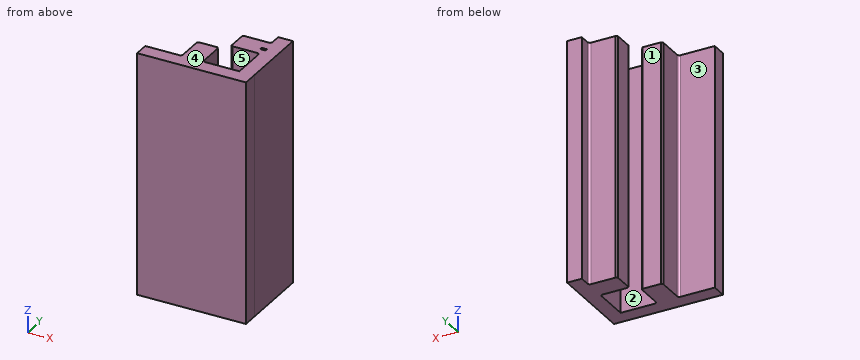
from build123d import *

# Parameters (mm, degrees)
BOSS_EXTRUDE1_DEPTH = 66.675
CUT_EXTRUDE1_REACH  = 75.8
CUT_EXTRUDE2_REACH  = 75.8
SKETCH5_W           = 1.489310624
SKETCH5_H           = 0.739469686
CUT_EXTRUDE3_DEPTH  = 2.54


with BuildPart() as part:
    # Sketch1 → Boss-Extrude1 (new body)
    with BuildSketch(Plane(origin=(0, 0, -3683), x_dir=(-1, 0, 0), z_dir=(0, 0, -1))):
        with BuildLine():
            Line((7.945265893, 3.588862728), (-1.198734107, 3.588862728))
            ThreePointArc((-1.198734107, 3.588862728), (-1.647746913, 3.774849922), (-1.833734107, 4.223862728))
            Line((-1.833734107, 4.223862728), (-1.833734107, 5.747862728))
            ThreePointArc((-1.833734107, 5.747862728), (-1.647746913, 6.196875535), (-1.198734107, 6.382862728))
            Line((-1.198734107, 6.382862728), (1.621629442, 6.382862728))
            Line((1.621629442, 6.382862728), (1.621629442, 6.890862686))
            Line((1.621629442, 6.890862686), (-2.214734107, 11.462862728))
            Line((-2.214734107, 11.462862728), (-7.294734107, 11.462862728))
            Line((-7.294734107, 11.462862728), (-11.131097656, 6.890862686))
            Line((-11.131097656, 6.890862686), (-11.131097656, 6.382862728))
            Line((-11.131097656, 6.382862728), (-8.310734107, 6.382862728))
            ThreePointArc((-8.310734107, 6.382862728), (-7.861721301, 6.196875535), (-7.675734107, 5.747862728))
            Line((-7.675734107, 5.747862728), (-7.675734107, 4.223862728))
            ThreePointArc((-7.675734107, 4.223862728), (-7.861721301, 3.774849922), (-8.310734107, 3.588862728))
            Line((-8.310734107, 3.588862728), (-17.454734107, 3.588862728))
            Line((-17.454734107, 3.588862728), (-17.727921752, 3.588862728))
            Line((-17.727921752, 3.588862728), (-17.727921752, 3.858842754))
            Line((-17.727921752, 3.858842754), (-17.728361466, 13.002372481))
            ThreePointArc((-17.728361466, 13.002372481), (-17.542256287, 13.451715967), (-17.092921752, 13.637842754))
            Line((-17.092921752, 13.637842754), (-15.568921752, 13.637842754))
            ThreePointArc((-15.568921752, 13.637842754), (-15.119908946, 13.45185556), (-14.933921752, 13.002842754))
            Line((-14.933921752, 13.002842754), (-14.933921752, 10.182479205))
            Line((-14.933921752, 10.182479205), (-14.425921794, 10.182479205))
            Line((-14.425921794, 10.182479205), (-9.853921752, 14.018842754))
            Line((-9.853921752, 14.018842754), (-9.853921752, 19.098842754))
            Line((-9.853921752, 19.098842754), (-14.425921794, 22.935206303))
            Line((-14.425921794, 22.935206303), (-14.933921752, 22.935206303))
            Line((-14.933921752, 22.935206303), (-14.933921752, 20.114842754))
            ThreePointArc((-14.933921752, 20.114842754), (-15.119908946, 19.665829948), (-15.568921752, 19.479842754))
            Line((-15.568921752, 19.479842754), (-17.092921752, 19.479842754))
            ThreePointArc((-17.092921752, 19.479842754), (-17.542476558, 19.66604812), (-17.728703542, 20.11559397))
            Line((-17.728703542, 20.11559397), (-17.728839138, 22.935206303))
            Line((-17.728839138, 22.935206303), (-21.787214199, 22.935206303))
            Line((-21.787214199, 22.935206303), (-21.791921752, 3.859128788))
            Line((-21.791921752, 3.859128788), (-21.791921752, 3.588862728))
            Line((-21.791921752, 3.588862728), (-21.791921752, -0.475137272))
            Line((-21.791921752, -0.475137272), (-17.727921752, -0.475137272))
            Line((-17.727921752, -0.475137272), (-17.454774021, -0.475137272))
            Line((-17.454774021, -0.475137272), (7.945225979, -0.475137272))
            Line((7.945225979, -0.475137272), (8.215492039, -0.475137272))
            Line((8.215492039, -0.475137272), (8.215492039, 3.588862728))
            Line((8.215492039, 3.588862728), (7.945265893, 3.588862728))
        make_face()
    extrude(amount=BOSS_EXTRUDE1_DEPTH)

    # Sketch2 → Cut-Extrude1 (cut, up to next)
    with BuildSketch(Plane.XY.offset(-3683), mode=Mode.PRIVATE) as cut_extrude1_sk1:
        with BuildLine():
            Line((11.131097656, 6.890862686), (11.131097656, 6.382862728))
            Line((11.131097656, 6.382862728), (8.310734107, 6.382862728))
            ThreePointArc((8.310734107, 6.382862728), (7.861721301, 6.196875535), (7.675734107, 5.747862728))
            Line((7.675734107, 5.747862728), (7.675734107, 11.00880461))
            Line((7.675734107, 11.00880461), (11.131097656, 6.890862686))
        make_face()
    cut_extrude1_tool1 = extrude(cut_extrude1_sk1.sketch, amount=-CUT_EXTRUDE1_REACH, mode=Mode.PRIVATE) & part.part
    # Sketch2 → Cut-Extrude1 (cut, up to next)
    with BuildSketch(Plane.XY.offset(-3683), mode=Mode.PRIVATE) as cut_extrude1_sk2:
        with BuildLine():
            Line((1.833734107, 5.747862728), (1.833734107, 11.00880461))
            Line((1.833734107, 11.00880461), (-1.621629442, 6.890862686))
            Line((-1.621629442, 6.890862686), (-1.621629442, 6.382862728))
            Line((-1.621629442, 6.382862728), (1.198734107, 6.382862728))
            ThreePointArc((1.198734107, 6.382862728), (1.647746913, 6.196875535), (1.833734107, 5.747862728))
        make_face()
    cut_extrude1_tool2 = extrude(cut_extrude1_sk2.sketch, amount=-CUT_EXTRUDE1_REACH, mode=Mode.PRIVATE) & part.part
    add(cut_extrude1_tool1.solids().sort_by_distance((8.930632, 7.925168, -3683))[0], mode=Mode.SUBTRACT)
    add(cut_extrude1_tool2.solids().sort_by_distance((0.578837, 7.925168, -3683))[0], mode=Mode.SUBTRACT)

    # Sketch3 → Cut-Extrude2 (cut, up to next)
    with BuildSketch(Plane.XY.offset(-3683), mode=Mode.PRIVATE) as cut_extrude2_sk1:
        with BuildLine():
            Line((15.568921752, 19.479842754), (10.307979871, 19.479842754))
            Line((10.307979871, 19.479842754), (14.425921794, 22.935206303))
            Line((14.425921794, 22.935206303), (14.933921752, 22.935206303))
            Line((14.933921752, 22.935206303), (14.933921752, 20.114842754))
            ThreePointArc((14.933921752, 20.114842754), (15.119908946, 19.665829948), (15.568921752, 19.479842754))
        make_face()
    cut_extrude2_tool1 = extrude(cut_extrude2_sk1.sketch, amount=-CUT_EXTRUDE2_REACH, mode=Mode.PRIVATE) & part.part
    # Sketch3 → Cut-Extrude2 (cut, up to next)
    with BuildSketch(Plane.XY.offset(-3683), mode=Mode.PRIVATE) as cut_extrude2_sk2:
        with BuildLine():
            Line((10.307979871, 13.637842754), (14.425921794, 10.182479205))
            Line((14.425921794, 10.182479205), (14.933921752, 10.182479205))
            Line((14.933921752, 10.182479205), (14.933921752, 13.002842754))
            ThreePointArc((14.933921752, 13.002842754), (15.119908946, 13.45185556), (15.568921752, 13.637842754))
            Line((15.568921752, 13.637842754), (10.307979871, 13.637842754))
        make_face()
    cut_extrude2_tool2 = extrude(cut_extrude2_sk2.sketch, amount=-CUT_EXTRUDE2_REACH, mode=Mode.PRIVATE) & part.part
    add(cut_extrude2_tool1.solids().sort_by_distance((13.391616, 20.73474, -3683))[0], mode=Mode.SUBTRACT)
    add(cut_extrude2_tool2.solids().sort_by_distance((13.391616, 12.382945, -3683))[0], mode=Mode.SUBTRACT)

    # Sketch5 → Cut-Extrude3 (cut)
    with BuildSketch(Plane.XY.offset(-3683)):
        with Locations((17.496622798, 16.016291439)):
            Rectangle(SKETCH5_W, SKETCH5_H)
    extrude(amount=-CUT_EXTRUDE3_DEPTH, mode=Mode.SUBTRACT)


solid = part.part
Verification items for the finished model (mm, model axes). Face numbers are marked on the shaded views. A direction names the side the tool comes from. Give positions to 0.01 mm unless a question says otherwise; leave off trailing zeros. Write each loop counter-clockwise with the first axis right and the second up, starting at its lowest first coordinate (ties: lowest second). Pieces come first, ordered by that corner, then holes.
(1) Access from +Z, -Z, +X, -X, +Y, -Y to the whole of each face (thin tool, end or side, straight path). Record for the marked faces 3, 4 and 5.
(2) Mould release check, pull along X, two halves, no side actions. Record for the marked faces 1 and 2: +X half, -X half, draft (parallel to the pull), parting line (faces both ways), or undercut.
(3) Gauge pin test, flat ends, axial feed: pin 1 (3 mm diameter, centred on y = 17, z = -3724, fed in from -X); pin 2 (10 mm diameter, centred on x = -4.5, z = -3693.5, fed in from +Y); pin 3 (5.5 mm diameter, centred on x = 3.5, z = -3725.5, fed in from +Y). Record the tip position at first contact, or that the pin passes through.
(4) Cross-section at A-A (y = 9.75). Enter the section's corners in (x, z) (3 decimals), plus the area to 3 significant figures.
(5) Cross-section at D-D (y = 21). Enter the section's corners in (x, z) (3 decimals).
(6) Material ranges on line 1 (X direction, y = 10.5, z = -3704); line 2 (Y direction, x = 11, z = -3735); line 3 (Y direction, x = -3.5, z = -3723), recorded low to high.
(7) Cross-section at C-C (x = 4.5). Enter the section's corners in (y, z) (3 decimals), plus the area to 3 significant figures.
Worked out:
1. face 3: +Z, -Z, -X, +Y
1. face 4: +Z, +X, -X, +Y, -Y
1. face 5: +Z, -Z, -X
2. face 1: draft
2. face 2: undercut
3. pin 1: stops at x = 9.85
3. pin 2: stops at y = 3.59
3. pin 3: stops at y = 11.46
4. outline: (1.834, -3749.675) - (7.676, -3749.675) - (7.676, -3683) - (1.834, -3683) - close; (17.728, -3749.675) - (21.79, -3749.675) - (21.79, -3683) - (17.728, -3683) - close
4. area: 660 mm2
5. outline: (17.729, -3749.675) - (21.788, -3749.675) - (21.788, -3683) - (17.729, -3683) - close
6. line 1: x = 1.83 to 7.68, 17.73 to 21.79
6. line 2: y = -0.48 to 3.59, 13.64 to 19.48
6. line 3: y = -0.48 to 3.59
7. outline: (-0.475, -3749.675) - (11.463, -3749.675) - (11.463, -3683) - (-0.475, -3683) - close
7. area: 796 mm2
